Autodesk Inventor part; units mm, degrees
ref_plane "YZ Plane" through (0, 0, 0) normal (1, 0, 0) x (0, 1, 0)
ref_plane "XZ Plane" through (0, 0, 0) normal (0, 1, 0) x (-1, 0, 0)
ref_plane "XY Plane" through (0, 0, 0) normal (0, 0, 1) x (1, 0, 0)
sketch "Skizze1" plane through (0, 0, 0) normal (0, 0, 1) x (1, 0, 0)
  circle A0 centre (0, 0) radius 6
  dimension "d0" = 12
extrude "Extrusion1" add sketch "Skizze1" along normal blind 35
sketch "Skizze2" plane through (0, 0, 0) normal (0, 0, -1) x (-1, 0, 0)
  circle A0 centre (0, 0) radius 4
  dimension "d3" = 8
extrude "Extrusion2" cut sketch "Skizze2" against normal blind 35
sketch "Skizze9" plane through (0, 0, 35) normal (0, 0, 1) x (1, 0, 0)
  arc A0 (0, 6) -> (-6, 0) centre (0, 0) ccw
  arc A1 (0, 4) -> (-4, 0) centre (0, 0) ccw
  line L0 (0, 4) -> (0, 6)
  line L1 (4, 0) -> (6, 0)
  line L2 (-4, 0) -> (-6, 0)
  arc A2 (0, -6) -> (6, 0) centre (0, 0) ccw
  arc A3 (0, -4) -> (4, 0) centre (0, 0) ccw
  line L3 (0, -4) -> (0, -6)
sketch "Skizze9 outline for Extrusion8" plane through (0, 0, 35) normal (0, 0, 1) x (1, 0, 0)
  line L0 (0, 6) -> (0, 4)
  arc A0 (0, 4) -> (-4, 0) centre (0, 0) ccw
  line L1 (-4, 0) -> (-6, 0)
  arc A1 (-6, 0) -> (0, 6) centre (0, 0) cw
  line L2 (4, 0) -> (6, 0)
  arc A2 (6, 0) -> (0, -6) centre (0, 0) cw
  line L3 (0, -6) -> (0, -4)
  arc A3 (0, -4) -> (4, 0) centre (0, 0) ccw
extrude "Extrusion8" add sketch "Skizze9 outline for Extrusion8" along normal blind 5
sketch "Skizze10" plane through (0, 0, 0) normal (0, 0, -1) x (-1, 0, 0)
  line L0 (0, -4) -> (0, -6)
  line L1 (-4, 0) -> (-6, 0)
  line L2 (-6, 0) -> (-4, 0)
  line L3 (0, 6) -> (0, 4)
  line L4 (0, -4) -> (0, -6)
  line L5 (-4, 0) -> (-6, 0)
  arc A0 (-6, 0) -> (0, -6) centre (0, 0) ccw
  arc A1 (6, 0) -> (0, 6) centre (0, 0) ccw
  arc A2 (4, 0) -> (0, 4) centre (0, 0) ccw
  line L6 (4, 0) -> (6, 0)
  line L7 (6, 0) -> (4, 0)
  arc A3 (-4, 0) -> (0, -4) centre (0, 0) ccw
extrude "Extrusion9" add sketch "Skizze10" along normal blind 5
properties part number "Steckhülse"
Here's how the part is built. I have some questions about the finished solid (model axes, mm). A direction names the side the tool comes from. Give positions to 0.01 mm unless a question says otherwise; leave off trailing zeros. Write each loop counter-clockwise with the first axis right and the second up, starting at its lowest first coordinate (ties: lowest second). Pieces come first, ordered by that corner, then holes. Notation, with made-up numbers: M -36.5,5.5 L -22.5,5.5 A22 ccw -22.5,13.5 Z; hole C 17.5,0 d10. An arc over 180 degrees is marked long. Put each result on its own line as item: value. Start each with the question number.
Item 1: If we section it at B-B, the plane y = 1.25: Write out the boundary of the cut face in (x, z), then the cut area to 3 significant figures.
Item 2: If we section it at D-D, the plane z = 19: Write out the boundary of the cut face in (x, y).
Item 3: If we section it at C-C, the plane x = 5: Write out the boundary of the cut face in (y, z), then the cut area to 3 significant figures.
Item 4: On a 3-axis mill with a long thin cutter (end or side, diameter ignored), from which of +Z, -Z, +X, -X, +Y, -Y can I reach the whole of each face in a straight line? I mean faces 1 (the flat face through (-5, 0, 37)), 2 (the flat face through (3, 3, 35)), 3 (the flat face through (-5, 0, -2)). Say none if no direction works.
Item 5: Will these pins go through, and if not, where does the flat tip stop? pin 1 (0.6 mm diameter, centred on x = 5, z = -2, fed in from +Y); pin 2 (1.5 mm diameter, centred on x = 1, z = 5.5, fed in from -Y); pin 3 (1.6 mm diameter, centred on y = 5.5, z = -1.5, fed in from +X); pin 4 (2 mm diameter, centred on x = 1.5, y = -2.5, fed in from -Z).
Item 6: If we section it at A-A, the plane z = 37: Write out the boundary of the cut face in (x, y), then the cut area to 3 significant figures.
Item 7: I need wall thicknesses on L1, parallel to X at y = 0, z = 25.5; L2, parallel to Z at x = -2.25, y = -5.5; L3, parallel to Y at x = 1.25, z = 16.5. Which ranges of each line are inside material? Lowest first, please. Write a range as from..to.
Values:
1. outline: M -5.87,-5 L -3.8,-5 L -3.8,40 L -5.87,40 Z; M 3.8,0 L 5.87,0 L 5.87,35 L 3.8,35 Z
1. area: 165 mm²
2. outline: C 0,0 d12; hole C 0,0 d8
3. outline: M -3.32,-5 L 0,-5 L 0,0 L 3.32,0 L 3.32,35 L 0,35 L 0,40 L -3.32,40 Z
3. area: 265 mm²
4. face 1: +Z, -X, -Y
4. face 2: +Z, +X, +Y
4. face 3: -Z, -X, -Y
5. pin 1: y = 0
5. pin 2: y = -5.99
5. pin 3: x = 0
5. pin 4: through
6. outline: M -6,0 L -4,0 A4 cw 0,4 L 0,6 A6 ccw Z; M 0,-6 A6 ccw 6,0 L 4,0 A4 cw 0,-4 Z
6. area: 31.4 mm²
7. L1: -6..-4, 4..6
7. L2: 0..35
7. L3: -5.87..-3.8, 3.8..5.87
